Can you work these out from the model? Positions are in its coordinate system, mm. Round coordinates to 2 decimals unless told otherwise and drop trailing zeros. Write each loop counter-clockwise with the first axis right and the second up, starting at its lowest first coordinate (ties: lowest second). Pieces come first, ordered by that corner, then holes. Notation, with made-up numbers: M 35,49 L 45,49 A19 cw 45,84 Z; hole C -14.5,78.5 d1. An arc over 180 degrees is marked long. Answer in a Markdown table with one row per item. Add a question column.
(1) Suppose I cut it at D-D, the plane z = -15. Write out the boundary of the cut face in (x, y), then the cut area to 3 significant figures.
(2) I'm going to push a flat-ended pin straight in: pin 1 (11 mm diameter, centred on y = 83.65, z = -15, fed in from +X). Where does the tip first touch, or does it pass through?
(3) Suppose I cut it at A-A, the plane y = -22.7. Write out the boundary of the cut face in (x, z), then the cut area to 3 significant figures.
(4) Suppose I cut it at B-B, the plane z = 0. Write out the boundary of the cut face in (x, y), then the cut area to 3 significant figures.
(5) If we mould it in two halves opening along Y, with no side actions, what happens to faces 1 (the face through (0, 90, 0)), 2 (the face through (0, -90, 0)), 3 (the face through (-0.089, -20.419, 15.454))? For each: released by +Y, released by -Y, zero draft, split by the parting line, or undercut.
(6) If I drill on probe 1 along Y at (x, z) = (-2.5, -15); probe 2 along Y at (x, z) = (0, -17.5); probe 3 along Y at (x, z) = (3, 14), over which ranges is the centre line in solid material (lowest first)?
(7) Suppose I cut it at C-C, the plane x = 4. Write out the boundary of the cut face in (y, z).
from build123d import *

# Parameters (mm, degrees)
CROQUIS1_W                    = 12.7
CROQUIS1_H                    = 180
SALIENTE_EXTRUIR1_DEPTH       = 25
TALADRO_ROSCADO_3_8_161_D     = 7.9375
TALADRO_DE_MARGEN_PARA_1_41_D = 6.7564
TALADRO_ROSCADO_1_4_281_D     = 5.4102


with BuildPart() as part:
    # Croquis1 → Saliente-Extruir1 (new, symmetric)
    with BuildSketch(Plane.XY):
        Rectangle(CROQUIS1_W, CROQUIS1_H)
    extrude(amount=SALIENTE_EXTRUIR1_DEPTH, both=True)

    # Taladro roscado 3/8-161 (through all)
    with Locations(Plane(origin=(6.35, 0, 0), x_dir=(0, 0, -1), z_dir=(1, 0, 0))):
        with Locations((0, -65)):
            Hole(TALADRO_ROSCADO_3_8_161_D / 2)

    # Taladro de margen para 1/41 (through all)
    with Locations(Plane.ZY.offset(6.35)):
        with Locations((-15, 83.65), (15, 83.65)):
            Hole(TALADRO_DE_MARGEN_PARA_1_41_D / 2)

    # Taladro roscado 1/4-281 (through all)
    with Locations(Plane(origin=(6.35, 0, 0), x_dir=(0, 0, -1), z_dir=(1, 0, 0))):
        with Locations((14, -22.7), (-14, -22.7)):
            Hole(TALADRO_ROSCADO_1_4_281_D / 2)


solid = part.part
Calculated:
| question | item | result |
|---|---|---|
| 1 | outline | M -6.35,-90 L 6.35,-90 L 6.35,-25.21 L -6.35,-25.21 Z; M -6.35,-20.19 L 6.35,-20.19 L 6.35,80.27 L -6.35,80.27 Z; M -6.35,87.03 L 6.35,87.03 L 6.35,90 L -6.35,90 Z |
| 1 | area | 2,140 mm² |
| 2 | pin 1 | x = 6.35 |
| 3 | outline | M -6.35,-25 L 6.35,-25 L 6.35,-16.71 L -6.35,-16.71 Z; M -6.35,-11.29 L 6.35,-11.29 L 6.35,11.29 L -6.35,11.29 Z; M -6.35,16.71 L 6.35,16.71 L 6.35,25 L -6.35,25 Z |
| 3 | area | 498 mm² |
| 4 | outline | M -6.35,-90 L 6.35,-90 L 6.35,-68.97 L -6.35,-68.97 Z; M -6.35,-61.03 L 6.35,-61.03 L 6.35,90 L -6.35,90 Z |
| 4 | area | 2,190 mm² |
| 5 | face 1 | released by +Y |
| 5 | face 2 | released by -Y |
| 5 | face 3 | undercut |
| 6 | probe 1 | -90 to -25.21, -20.19 to 80.27, 87.03 to 90 |
| 6 | probe 2 | -90 to 81.38, 85.92 to 90 |
| 6 | probe 3 | -90 to -25.41, -19.99 to 80.42, 86.88 to 90 |
| 7 | outline | M -90,-25 L 90,-25 L 90,25 L -90,25 Z; hole C -65,0 d7.94; hole C -22.7,-14 d5.41; hole C -22.7,14 d5.41; hole C 83.65,-15 d6.76; hole C 83.65,15 d6.76 |
